The model under review builds one solid part; all positions refer to its coordinate system, in mm. Coordinates: 2 decimals unless noted, no trailing zeros. Write each loop counter-clockwise with the first axis right and the second up, starting at its lowest first coordinate (ties: lowest second). Pieces come first, ordered by that corner, then holes. Notation, with made-up numbers: (-28.75, 39.5) - (16.25, 39.5) arc R16 ccw to (16.25, 49.5) - close; hole circle Ø9 at (29.25, 59). An arc over 180 degrees is marked (long way). Put each result on its own line as item: value. Start each with the question number.
Item 1: For pin 1 (5 mm diameter, centred on x = -7, z = -3, fed in from -Y); pin 2 (4 mm diameter, centred on x = 0, y = -0.25, fed in from -Z); pin 3 (1.5 mm diameter, centred on x = -5, z = -2, fed in from -Y), all flat-tipped, find the tip position at first contact; note any pin that passes through.
Item 2: Consider section B-B on y = 0. Give the boundary of the cut face in (x, z) (3 decimals), then the cut area to 3 significant figures.
Item 3: Consider section D-D on x = 5. Give the boundary of the cut face in (y, z) (3 decimals).
Item 4: To check wall thickness, follow L1, parallel to X at y = -0.25, z = 1.75 (3 decimals); L2, parallel to X at y = 1, z = 2.5 (3 decimals); L3, parallel to Y at x = 0, z = 0.5. State the ranges of each line that lie inside material, in increasing order. Write a range as [from, to].
Item 5: Consider section C-C on x = 0. Give the boundary of the cut face in (y, z) (3 decimals), then the cut area to 3 significant figures.
Item 6: Mouldability with a two-part tool opening along X and no side actions: class faces 1 (the face through (1.844, 2.642, 0.068)), 2 (the face through (-9.525, 0, 0)), 3 (the face through (9.525, 0, 0)) as pulls with the +X half, pulls with the -X half, needs draft (parallel to the pull), parting line crosses it, or undercut.
Item 7: Consider section A-A on z = 0. Give the boundary of the cut face in (x, y) (3 decimals), then the cut area to 3 significant figures.
```python
from build123d import *

# Parameters (mm, degrees)
ESQUISSE1_R             = 4.765
BOSS_EXTRU_1_DEPTH      = 9.525
CHANFREIN1_SIZE         = 0.76
ESQUISSE2_R             = 3.43
ENL_V_MAT_EXTRU_1_DEPTH = 9.525


with BuildPart() as part:
    # Esquisse1 → Boss.-Extru.1 (new body, symmetric)
    with BuildSketch(Plane(origin=(0, 0, 0), x_dir=(0, 0, -1), z_dir=(1, 0, 0))):
        Circle(ESQUISSE1_R)
    extrude(amount=BOSS_EXTRU_1_DEPTH, both=True)

    # Chanfrein1
    chanfrein1_edges = [part.edges().sort_by_distance(p)[0] for p in [
        (-9.525, 0, 4.765),
        (9.525, 0, 4.765),
    ]]
    chamfer(chanfrein1_edges, length=CHANFREIN1_SIZE)

    # Esquisse2 → Enlèv. mat.-Extru.1 (cut, symmetric)
    with BuildSketch(Plane.XY):
        with Locations((0, -0.25)):
            Circle(ESQUISSE2_R)
    extrude(amount=ENL_V_MAT_EXTRU_1_DEPTH, both=True, mode=Mode.SUBTRACT)


solid = part.part
```
Report:
1. pin 1: y = -4.74
1. pin 2: through
1. pin 3: y = -4.6
2. outline: (-9.525, -4.005) - (-8.765, -4.765) - (-3.421, -4.765) - (-3.421, 4.765) - (-8.765, 4.765) - (-9.525, 4.005) - close; (3.421, -4.765) - (8.765, -4.765) - (9.525, -4.005) - (9.525, 4.005) - (8.765, 4.765) - (3.421, 4.765) - close
2. area: 115 mm²
3. outline: circle Ø9.53 at (0, 0)
4. L1: [-9.525, -3.43], [3.43, 9.525]
4. L2: [-9.525, -3.194], [3.194, 9.525]
4. L3: [-4.74, -3.68], [3.18, 4.74]
5. outline: (-3.68, -3.027) - (-3.68, 3.027) arc R4.765 ccw to start; (3.18, -3.549) arc R4.765 ccw to (3.18, 3.549) - close
5. area: 12.3 mm²
6. face 1: undercut
6. face 2: pulls with the -X half
6. face 3: pulls with the +X half
7. outline: (-9.525, -4.005) - (-8.765, -4.765) - (8.765, -4.765) - (9.525, -4.005) - (9.525, 4.005) - (8.765, 4.765) - (-8.765, 4.765) - (-9.525, 4.005) - close; hole circle Ø6.86 at (0, -0.25)
7. area: 143 mm²
